Geometry check sheet. Reference: the model listing, model coordinates, mm. A direction names the side the tool comes from. Give positions to 0.01 mm unless a question says otherwise; leave off trailing zeros. Write each loop counter-clockwise with the first axis right and the second up, starting at its lowest first coordinate (ties: lowest second). Pieces come first, ordered by that corner, then holes. Notation, with made-up numbers: (28.25, 5) - (81.25, 5) arc R28 ccw to (81.25, 29) - close; hole circle Ø8 at (31.5, 30). An arc over 180 degrees is marked (long way). Write item = value, one per line. Start each with the question number.
(1) Depth check by flat-ended pin: pin 1 Ø3 at (y, z) = (-10, -10) entering from -X; pin 2 Ø2 at (y, z) = (-10, 10) entering from +X; pin 3 Ø6 at (y, z) = (-3, -1) entering from -X. Enter the tip coordinate at first touch or a pass-through.
(2) Section check B-B, the plane x = 3.5. Enter the section's corners in (y, z).
(3) Draft check along Y on faces 4 (the conical face through (4.88, -9.92, -9.8)), 5 (the flat face through (6, 22.7, 0)), 6 (the flat face through (2, 0, 6)), 7 (the cylindrical face through (7.72, 9.95, -8.75)). Enter one of: pulls with the +Y half, pulls with the -Y half, needs draft (parallel to the pull), parting line crosses it, or undercut.
(4) Access from +Z, -Z, +X, -X, +Y, -Y to the whole of each face (thin tool, end or side, straight path). Record for faces 1 (the cylindrical face through (7.719, -10.845, -9.079)), 2 (the flat face through (2, 0, -6)), 3 (the flat face through (5, 0, -13.5)).
(5) Section check C-C, the plane y = 3. Enter the section's corners in (x, z), plus the area to 3 significant figures.
(6) Section check A-A, the plane x = 7.75. Enter the section's corners in (y, z), plus the area to 3 significant figures.
(7) Thickness scan on L1, parallel to Z at x = 8.2, y = 10; L2, parallel to Y at x = 8.45, z = 10; L3, parallel to Z at x = 2, y = -15.5. Record the ranges inside material, lowest first.
```python
from build123d import *

# Parameters (mm, degrees)
SKETCH_1_W             = 27
SKETCH_1_H             = 45.4
EXTRUDE_1_DEPTH        = 10
SKETCH_2_W             = 5
SKETCH_2_H             = 12
CUT_EXTRUDE_1_DEPTH    = 49.408780195
HOLE_WIZARD_M3_1_D     = 2.5
HOLE_WIZARD_M3_1_DEPTH = 4.5
HOLE_WIZARD_M3_1_TIP   = 0.751075774


with BuildPart() as part:
    # 草圖1 → 伸長1 (new body)
    with BuildSketch(Plane(origin=(0, 0, 0), x_dir=(0, 0, -1), z_dir=(1, 0, 0))):
        Rectangle(SKETCH_1_W, SKETCH_1_H)
    extrude(amount=EXTRUDE_1_DEPTH)

    # 草圖2 → 除料-伸長1 (cut, through all)
    with BuildSketch(Plane.XZ.offset(22.7)):
        with Locations((2.5, 0)):
            Rectangle(SKETCH_2_W, SKETCH_2_H)
    extrude(amount=-CUT_EXTRUDE_1_DEPTH, mode=Mode.SUBTRACT)

    # M3 螺紋孔1
    with Locations(Plane(origin=(10, 10, -10), x_dir=(0, 0, 1), z_dir=(1, 0, 0))):
        with Locations((0, 0), (0, 20), (20, 0), (20, 20)):
            Hole(HOLE_WIZARD_M3_1_D / 2, depth=HOLE_WIZARD_M3_1_DEPTH)
            with Locations((0, 0, -(HOLE_WIZARD_M3_1_DEPTH + HOLE_WIZARD_M3_1_TIP / 2))):  # 118° drill point
                Cone(0, HOLE_WIZARD_M3_1_D / 2, HOLE_WIZARD_M3_1_TIP, mode=Mode.SUBTRACT)


solid = part.part
```
Model answer:
q1.pin_1 = 0
q1.pin_2 = 5.35
q1.pin_3 = 5
q2.outline = (-22.7, -13.5) - (22.7, -13.5) - (22.7, -6) - (-22.7, -6) - close; (-22.7, 6) - (22.7, 6) - (22.7, 13.5) - (-22.7, 13.5) - close
q3.face_4 = undercut
q3.face_5 = pulls with the +Y half
q3.face_6 = needs draft
q3.face_7 = undercut
q4.face_1 = +X
q4.face_2 = -X, +Y, -Y
q4.face_3 = -Z, +X, -X, +Y, -Y
q5.outline = (0, -13.5) - (10, -13.5) - (10, 13.5) - (0, 13.5) - (0, 6) - (5, 6) - (5, -6) - (0, -6) - close
q5.area = 210 mm²
q6.outline = (-22.7, -13.5) - (22.7, -13.5) - (22.7, 13.5) - (-22.7, 13.5) - close; hole circle Ø2.5 at (-10, -10); hole circle Ø2.5 at (-10, 10); hole circle Ø2.5 at (10, -10); hole circle Ø2.5 at (10, 10)
q6.area = 1,210 mm²
q7.L1 = -13.5 to -11.25, -8.75 to 8.75, 11.25 to 13.5
q7.L2 = -22.7 to -11.25, -8.75 to 8.75, 11.25 to 22.7
q7.L3 = -13.5 to -6, 6 to 13.5
